Drawing for the job (mm, zero at the part's lowest x, y, z). Coordinates: 2 decimals unless noted, no trailing zeros. Order: outer loops, then holes, each group sorted by start corner. A loop starts at its lowest first (then second) coordinate and runs counter-clockwise, first axis right, second up.
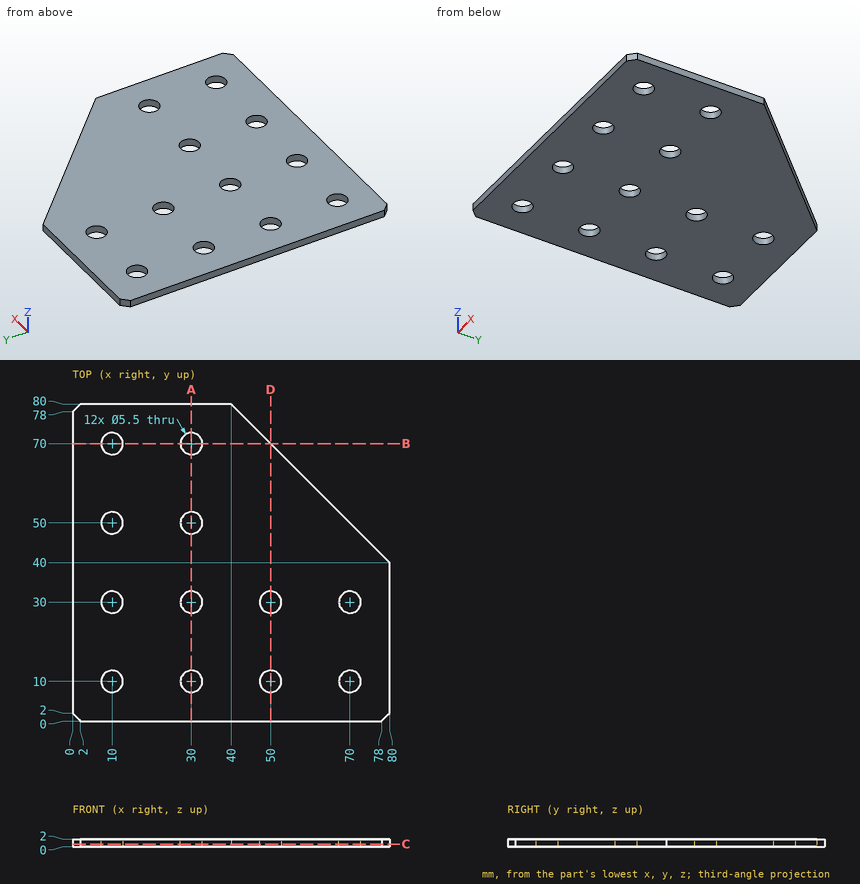
1) Pin check, flat tip, straight feed: P1, Ø4.5, axis at x = 50, y = 30, coming from the -Z side (3 decimals). Stop position of the tip, or through.
2) Slice it at D-D (x = 50). List the corners of the cut face in (y, z), plus the area to 3 significant figures.
3) Slice it at A-A (x = 30). List the corners of the cut face in (y, z), plus the area to 3 significant figures.
4) Drill centre lines: probe 1 along Y at (x, z) = (10, 0.6); probe 2 along X at (y, z) = (29, 1.55). Where is each one in solid material? Low to high.
5) Slice it at B-B (y = 70). List the corners of the cut face in (x, z).
6) Slice it at C-C (z = 0.7). Give the number of separate pieces and of enclosed holes in the cut face, plus the area to 3 significant figures.
Worked out:
1. P1: passes through
2. outline: (0, 0) - (7.25, 0) - (7.25, 2) - (0, 2) - close; (12.75, 0) - (27.25, 0) - (27.25, 2) - (12.75, 2) - close; (32.75, 0) - (70, 0) - (70, 2) - (32.75, 2) - close
2. area: 118 mm2
3. outline: (0, 0) - (7.25, 0) - (7.25, 2) - (0, 2) - close; (12.75, 0) - (27.25, 0) - (27.25, 2) - (12.75, 2) - close; (32.75, 0) - (47.25, 0) - (47.25, 2) - (32.75, 2) - close; (52.75, 0) - (67.25, 0) - (67.25, 2) - (52.75, 2) - close; (72.75, 0) - (80, 0) - (80, 2) - (72.75, 2) - close
3. area: 116 mm2
4. probe 1: y = 0 to 7.25, 12.75 to 27.25, 32.75 to 47.25, 52.75 to 67.25, 72.75 to 80
4. probe 2: x = 0 to 7.44, 12.56 to 27.44, 32.56 to 47.44, 52.56 to 67.44, 72.56 to 80
5. outline: (0, 0) - (7.25, 0) - (7.25, 2) - (0, 2) - close; (12.75, 0) - (27.25, 0) - (27.25, 2) - (12.75, 2) - close; (32.75, 0) - (50, 0) - (50, 2) - (32.75, 2) - close
6. separate pieces: 1
6. enclosed holes: 12
6. area: 5,310 mm2
